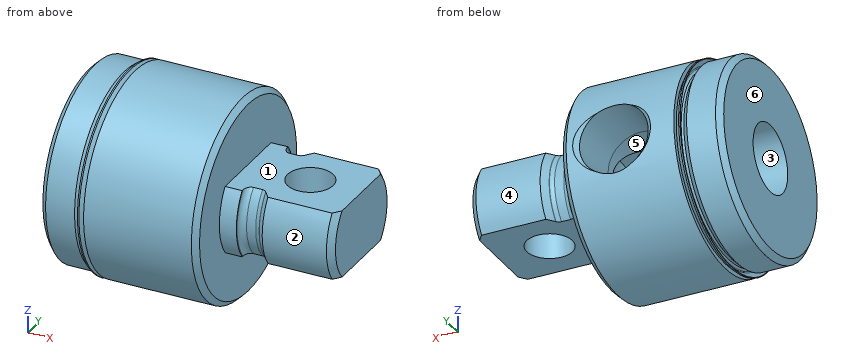
Autodesk Inventor part; units mm, degrees
ref_plane "1_XY" through (24.6126, 0, 0) normal (1, 0, 0) x (0, 0, -1)
ref_plane "1_YZ" through (24.6126, 0, 0) normal (0, 0, -1) x (0, 1, 0)
ref_plane "1_ZX" through (24.6126, 0, 0) normal (0, 1, 0) x (1, 0, 0)
sketch "Sketch_18" plane through (0, 0, 0) normal (0, 0, 1) x (1, 0, 0)
  line L0 (22.225, 0) -> (0, 0)
  line L1 (0, 0) -> (0, 12.846)
  line L2 (0, 12.846) -> (0.762, 13.6081)
  line L3 (0.762, 13.6081) -> (4.826, 13.6081)
  line L4 (4.826, 13.6081) -> (5.588, 12.846)
  line L5 (5.588, 12.846) -> (6.35, 12.846)
  line L6 (6.35, 12.846) -> (6.35, 14.1097)
  line L7 (6.35, 14.1097) -> (21.463, 14.1097)
  line L8 (21.463, 14.1097) -> (22.225, 13.3477)
  line L9 (22.225, 13.3477) -> (22.225, 0)
  line L10 (22.225, 0) -> (0, 0)
revolve "Revolution1" add sketch "Sketch_18" angle 360 about axis through (22.225, 0, 0) along (1, 0, 0)
sketch "Sketch_15" plane through (0, 0, 0) normal (0, 0, 1) x (1, 0, 0)
  line L0 (38.1, 0) -> (22.225, 0)
  line L1 (22.225, 0) -> (22.225, 7.9057)
  line L2 (22.225, 7.9057) -> (24.6126, 7.9057)
  line L3 (24.6126, 7.9057) -> (24.6126, 7.7279)
  arc A0 (24.6126, 7.7279) -> (25.5016, 6.839) centre (25.5016, 7.7279) ccw
  line L4 (25.5016, 6.839) -> (26.7843, 6.839)
  arc A1 (26.7843, 6.839) -> (27.383, 7.0708) centre (26.7843, 7.7279) ccw
  line L5 (27.383, 7.0708) -> (27.4129, 7.098)
  line L6 (27.4129, 7.098) -> (28.2524, 7.9375)
  line L7 (28.2524, 7.9375) -> (37.2605, 7.9375)
  line L8 (37.2605, 7.9375) -> (38.1, 7.098)
  line L9 (38.1, 7.098) -> (38.1, 0)
  line L10 (38.1, 0) -> (22.225, 0)
revolve "Revolution2" add sketch "Sketch_15" angle 360 about axis through (38.1, 0, 0) along (1, 0, 0)
thread "Thread1"
sketch "Sketch_9" plane through (38.1, 0, 0) normal (1, 0, 0) x (0, 0, -1)
  line L0 (-28.2194, -56.4388) -> (28.2194, -56.4388)
  line L1 (28.2194, -56.4388) -> (28.2194, 56.4388)
  line L2 (28.2194, 56.4388) -> (-28.2194, 56.4388)
  line L3 (-28.2194, 56.4388) -> (-28.2194, -56.4388)
  line L4 (-4.7307, -28.2194) -> (4.7307, -28.2194)
  line L5 (4.7307, -28.2194) -> (4.7307, 28.2194)
  line L6 (4.7307, 28.2194) -> (-4.7307, 28.2194)
  line L7 (-4.7307, 28.2194) -> (-4.7307, -28.2194)
extrude "Extrusion1" cut sketch "Sketch_9" against normal blind 15.875
sketch "Sketch4" plane through (0, 0, 0) normal (-1, 0, 0) x (0, 0, 1)
  point P0 (0, 0)
hole "Hole1" at (0, 0, 0) direction (1, 0, 0) diameter 9.525 depth 20.955 tip angle 120
sketch "Sketch_47" plane through (0, 0, 0) normal (0, 0, 1) x (1, 0, 0)
  line L0 (15.0876, 0) -> (15.0876, 14.1097)
  line L1 (15.0876, 14.1097) -> (20.5423, 14.1097)
  line L2 (20.5423, 14.1097) -> (19.9073, 13.4747)
  line L3 (19.9073, 13.4747) -> (19.6754, 6.0491)
  line L4 (19.6754, 6.0491) -> (19.6754, 0)
  line L5 (19.6754, 0) -> (15.0876, 0)
  line L6 (15.0876, 0) -> (15.0876, 14.1097)
revolve "Revolution3" cut sketch "Sketch_47" angle 360 about axis through (15.0876, 0, 0) along (0, -1, 0)
thread "Thread2"
sketch "Sketch_24" plane through (0, 0, 0) normal (0, 0, 1) x (1, 0, 0)
  line L0 (6.35, 0) -> (5.588, 0)
  line L1 (5.4861, 14.1097) -> (5.4861, 14.0255)
  line L2 (5.4861, 14.0255) -> (6.2275, 13.2842)
  arc A0 (6.2275, 13.1046) -> (6.2275, 13.2842) centre (6.1377, 13.1944) ccw
  line L3 (6.2275, 13.1046) -> (5.969, 12.846)
  line L4 (5.969, 12.846) -> (5.588, 12.846)
  line L5 (5.588, 12.846) -> (5.588, 12.5921)
  line L6 (5.588, 12.5921) -> (6.35, 12.5921)
  line L7 (6.35, 12.5921) -> (6.35, 13.449)
  line L8 (6.35, 13.449) -> (5.6893, 14.1097)
  line L9 (5.6893, 14.1097) -> (5.4861, 14.1097)
revolve "Revolution4" add sketch "Sketch_24" angle 360 about axis through (6.35, 0, 0) along (1, 0, 0)
sketch "Sketch_43" plane through (0, 0, 0) normal (0, 0, 1) x (1, 0, 0)
  circle A0 centre (30.9626, 0) radius 3.2004
extrude "Extrusion2" cut sketch "Sketch_43" along normal mid plane 14.1922
ref_plane "1_XY" through (24.6126, 0, 0) normal (1, 0, 0) x (0, 0, -1)
ref_plane "1_YZ" through (24.6126, 0, 0) normal (0, 0, -1) x (0, 1, 0)
ref_plane "1_ZX" through (24.6126, 0, 0) normal (0, 1, 0) x (1, 0, 0)
ref_plane "c1_XY" through (22.225, 7.9057, 0) normal (0, 0, 1) x (1, 0, 0)
ref_plane "c1_YZ" through (22.225, 7.9057, 0) normal (1, 0, 0) x (0, 1, 0)
ref_plane "c1_ZX" through (22.225, 7.9057, 0) normal (0, 1, 0) x (0, 0, 1)
ref_plane "c2_XY" through (22.225, -7.9057, 0) normal (0, 0, 1) x (1, 0, 0)
ref_plane "c2_YZ" through (22.225, -7.9057, 0) normal (1, 0, 0) x (0, 1, 0)
ref_plane "c2_ZX" through (22.225, -7.9057, 0) normal (0, 1, 0) x (0, 0, 1)
ref_plane "cc1_XY" through (22.225, 0, 0) normal (0, 0, 1) x (1, 0, 0)
ref_plane "cc1_YZ" through (22.225, 0, 0) normal (1, 0, 0) x (0, 1, 0)
ref_plane "cc1_ZX" through (22.225, 0, 0) normal (0, 1, 0) x (0, 0, 1)
ref_plane "cc2_XY" through (24.6126, 0, 0) normal (0, 0, 1) x (1, 0, 0)
ref_plane "cc2_YZ" through (24.6126, 0, 0) normal (1, 0, 0) x (0, 1, 0)
ref_plane "cc2_ZX" through (24.6126, 0, 0) normal (0, 1, 0) x (0, 0, 1)
ref_plane "lovra1_XY" through (33.3248, 0, 0) normal (1, 0, 0) x (0, 0, -1)
ref_plane "lovra1_YZ" through (33.3248, 0, 0) normal (0, 0, -1) x (0, 1, 0)
ref_plane "lovra1_ZX" through (33.3248, 0, 0) normal (0, 1, 0) x (1, 0, 0)
ref_plane "lovra2_XY" through (33.3248, 11.049, 0) normal (1, 0, 0) x (0, 0, -1)
ref_plane "lovra2_YZ" through (33.3248, 11.049, 0) normal (0, 0, -1) x (0, 1, 0)
ref_plane "lovra2_ZX" through (33.3248, 11.049, 0) normal (0, 1, 0) x (1, 0, 0)
ref_plane "lovra21_XY" through (0, 0, 5.2705) normal (1, 0, 0) x (0, 0, -1)
ref_plane "lovra21_YZ" through (0, 0, 5.2705) normal (0, 0, -1) x (0, 1, 0)
ref_plane "lovra21_ZX" through (0, 0, 5.2705) normal (0, 1, 0) x (1, 0, 0)
ref_plane "lovra22_XY" through (0, 0, -5.2705) normal (1, 0, 0) x (0, 0, -1)
ref_plane "lovra22_YZ" through (0, 0, -5.2705) normal (0, 0, -1) x (0, 1, 0)
ref_plane "lovra22_ZX" through (0, 0, -5.2705) normal (0, 1, 0) x (1, 0, 0)
ref_plane "lovra3_XY" through (33.3248, -11.049, 0) normal (1, 0, 0) x (0, 0, -1)
ref_plane "lovra3_YZ" through (33.3248, -11.049, 0) normal (0, 0, -1) x (0, 1, 0)
ref_plane "lovra3_ZX" through (33.3248, -11.049, 0) normal (0, 1, 0) x (1, 0, 0)
ref_plane "olen_XY" through (30.9626, 0, 0) normal (1, 0, 0) x (0, 0, -1)
ref_plane "olen_YZ" through (30.9626, 0, 0) normal (0, 0, -1) x (0, 1, 0)
ref_plane "olen_ZX" through (30.9626, 0, 0) normal (0, 1, 0) x (1, 0, 0)
ref_plane "p1_XY" through (38.1, 0, 4.7307) normal (1, 0, 0) x (0, 0, -1)
ref_plane "p1_YZ" through (38.1, 0, 4.7307) normal (0, 0, -1) x (0, 1, 0)
ref_plane "p1_ZX" through (38.1, 0, 4.7307) normal (0, 1, 0) x (1, 0, 0)
ref_plane "p2_XY" through (38.1, 0, -4.7307) normal (1, 0, 0) x (0, 0, -1)
ref_plane "p2_YZ" through (38.1, 0, -4.7307) normal (0, 0, -1) x (0, 1, 0)
ref_plane "p2_ZX" through (38.1, 0, -4.7307) normal (0, 1, 0) x (1, 0, 0)
ref_plane "port_XY" through (15.0876, 14.1097, 0) normal (0, 0, 1) x (1, 0, 0)
ref_plane "port_YZ" through (15.0876, 14.1097, 0) normal (1, 0, 0) x (0, 1, 0)
ref_plane "port_ZX" through (15.0876, 14.1097, 0) normal (0, 1, 0) x (0, 0, 1)
ref_plane "port2_XY" through (38.1, 0, 0) normal (1, 0, 0) x (0, 0, -1)
ref_plane "port2_YZ" through (38.1, 0, 0) normal (0, 0, -1) x (0, 1, 0)
ref_plane "port2_ZX" through (38.1, 0, 0) normal (0, 1, 0) x (1, 0, 0)
ref_plane "thd1_XY" through (38.1, 0, 7.9375) normal (1, 0, 0) x (0, 0, -1)
ref_plane "thd1_YZ" through (38.1, 0, 7.9375) normal (0, 0, -1) x (0, 1, 0)
ref_plane "thd1_ZX" through (38.1, 0, 7.9375) normal (0, 1, 0) x (1, 0, 0)
ref_plane "thd2_XY" through (38.1, 0, -7.9375) normal (1, 0, 0) x (0, 0, -1)
ref_plane "thd2_YZ" through (38.1, 0, -7.9375) normal (0, 0, -1) x (0, 1, 0)
ref_plane "thd2_ZX" through (38.1, 0, -7.9375) normal (0, 1, 0) x (1, 0, 0)
ref_plane "to_mounting_bracket_XY" through (22.225, 0, 0) normal (1, 0, 0) x (0, 0, -1)
ref_plane "to_mounting_bracket_YZ" through (22.225, 0, 0) normal (0, 0, -1) x (0, 1, 0)
ref_plane "to_mounting_bracket_ZX" through (22.225, 0, 0) normal (0, 1, 0) x (1, 0, 0)
ref_plane "to_nut_XY" through (24.6126, 0, 0) normal (1, 0, 0) x (0, 0, -1)
ref_plane "to_nut_YZ" through (24.6126, 0, 0) normal (0, 0, -1) x (0, 1, 0)
ref_plane "to_nut_ZX" through (24.6126, 0, 0) normal (0, 1, 0) x (1, 0, 0)
ref_plane "to_pin_XY" through (30.9626, 0, 0) normal (0, 0, 1) x (1, 0, 0)
ref_plane "to_pin_YZ" through (30.9626, 0, 0) normal (1, 0, 0) x (0, 1, 0)
ref_plane "to_pin_ZX" through (30.9626, 0, 0) normal (0, 1, 0) x (0, 0, 1)
ref_plane "to_screw_XY" through (15.0876, -7.0612, -10.2743) normal (0, 0, -1) x (1, 0, 0)
ref_plane "to_screw_YZ" through (15.0876, -7.0612, -10.2743) normal (1, 0, 0) x (0, -1, 0)
ref_plane "to_screw_ZX" through (15.0876, -7.0612, -10.2743) normal (0, -1, 0) x (0, 0, -1)
ref_plane "to_tube_XY" through (5.588, 0, 0) normal (1, 0, 0) x (0, 0, -1)
ref_plane "to_tube_YZ" through (5.588, 0, 0) normal (0, 0, -1) x (0, 1, 0)
ref_plane "to_tube_ZX" through (5.588, 0, 0) normal (0, 1, 0) x (1, 0, 0)
properties part number "09P0K000_rear_head"
The model under review builds one solid part; all positions refer to its coordinate system, in mm. Face numbers are marked on the shaded views. A direction names the side the tool comes from. Coordinates: 2 decimals unless noted, no trailing zeros. Write each loop counter-clockwise with the first axis right and the second up, starting at its lowest first coordinate (ties: lowest second). Pieces come first, ordered by that corner, then holes. Notation, with made-up numbers: (4.25, 88.25) - (42.25, 88.25) arc R27 cw to (42.25, 127.25) - close; hole circle Ø11 at (83, 18.25). An arc over 180 degrees is marked (long way). Answer in a Markdown table with one row per item. Add a question column.
Q1. Consider section A-A on x = 4. Give the boundary of the cut face in (y, z) (1 decimal).
Q2. Consider section B-B on z = -2. Give the number of separate pieces and of enclosed holes in the cut face, then the cut area to 3 significant figures.
Q3. Draft analysis for pull direction Z (two halves, no side actions). For the marked faces 4, 5 and 6, state which applies: +Z half, -Z half, draft (parallel to the pull), parting line (faces both ways), or undercut.
Q4. To check wall thickness, follow line 1 along X through (y, z) = (-7.75, 3.5) (3 decimals); line 2 along Z through (x, y) = (30, -5.5); line 3 along Z through (x, y) = (13.5, 9.5). State the ranges of each line that lie inside material, in increasing order. Write a range as from..to.
Q5. Clearance check with flat-ended pins moving along their axes: pin 1 (1 mm diameter, centred on x = 22.5, z = -6, fed in from +Y); pin 2 (3 mm diameter, centred on y = 8, z = 1, fed in from -X); pin 3 (2 mm diameter, centred on x = 10, y = 8, fed in from -Z); pin 4 (10 mm diameter, centred on x = 19.5, z = 7, fed in from -Y). State where each tip first meets the part, or that it passes through.
Q6. For the marked faces 1, 2 and 3, list the 3-axis set-ups (+Z, -Z, +X, -X, +Y, -Y) from which the entire face can be reached by the end or side of a thin tool; tool diameter is ignored.
Answers below:
| question | item | result |
|---|---|---|
| 1 | outline | circle Ø27.2 at (0, 0); hole circle Ø9.5 at (0, 0) |
| 2 | separate pieces | 2 |
| 2 | enclosed holes | 1 |
| 2 | area | 545 mm² |
| 3 | face 4 | parting line |
| 3 | face 5 | undercut |
| 3 | face 6 | draft |
| 4 | line 1 | 0..22.225 |
| 4 | line 2 | -4.73..4.73 |
| 4 | line 3 | -10.43..-4.42, 4.42..10.43 |
| 5 | pin 1 | y = 12.22 |
| 5 | pin 2 | x = 0 |
| 5 | pin 3 | z = -12.25 |
| 5 | pin 4 | y = -13.97 |
| 6 | face 1 | +Z, +X, +Y, -Y |
| 6 | face 2 | +X, -Y |
| 6 | face 3 | -X |
